Could you check a few things on this model? Use its own coordinates, in mm. Face numbers are marked on the shaded views. A direction names the side the tool comes from. Coordinates: 2 decimals unless noted, no trailing zeros. Order: outer loops, then holes, each group sorted by start corner. A loop starts at its lowest first (then second) coordinate and runs counter-clockwise, first axis right, second up.
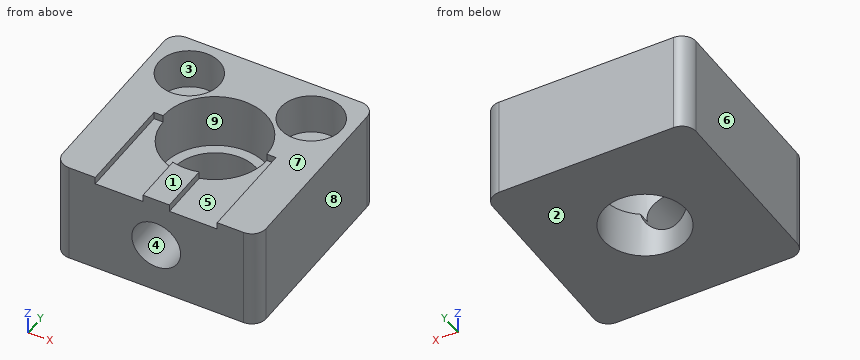
```python
from build123d import *

# Parameters (mm, degrees)
SKETCH1_W           = 10
SKETCH1_H           = 5
BOSS_EXTRUDE1_DEPTH = 10
SKETCH2_R           = 2.05
CUT_EXTRUDE1_DEPTH  = 16
SKETCH3_R           = 2.55
CUT_EXTRUDE2_DEPTH  = 2.7
SKETCH5_W           = 2.35
SKETCH5_H           = 0.35
CUT_EXTRUDE3_DEPTH  = 5
SKETCH6_R           = 1.5
CUT_EXTRUDE4_DEPTH  = 2
SKETCH8_R           = 1.2
CUT_EXTRUDE5_DEPTH  = 3.5
FILLET1_R           = 0.7


with BuildPart() as part:
    # Sketch1 → Boss-Extrude1 (new body)
    with BuildSketch(Plane(origin=(0, 0, 0), x_dir=(1, 0, 0), z_dir=(0, 1, 0))):
        with Locations((5, 2.5)):
            Rectangle(SKETCH1_W, SKETCH1_H)
    extrude(amount=BOSS_EXTRUDE1_DEPTH)

    # Sketch2 → Cut-Extrude1 (cut, through all)
    with BuildSketch(Plane.XY):
        with Locations((5, 5)):
            Circle(SKETCH2_R)
    extrude(amount=-CUT_EXTRUDE1_DEPTH, mode=Mode.SUBTRACT)

    # Sketch3 → Cut-Extrude2 (cut)
    with BuildSketch(Plane.XY):
        with Locations((5, 5)):
            Circle(SKETCH3_R)
    extrude(amount=-CUT_EXTRUDE2_DEPTH, mode=Mode.SUBTRACT)

    # Sketch5 → Cut-Extrude3 (cut)
    with BuildSketch(Plane.XZ):
        with Locations((3.175, -0.175)):
            Rectangle(SKETCH5_W, SKETCH5_H)
        with Locations((6.825, -0.175)):
            Rectangle(SKETCH5_W, SKETCH5_H)
    extrude(amount=-CUT_EXTRUDE3_DEPTH, mode=Mode.SUBTRACT)

    # Sketch6 → Cut-Extrude4 (cut)
    with BuildSketch(Plane.XY):
        with Locations((2, 8)):
            Circle(SKETCH6_R)
        with Locations((8, 8)):
            Circle(SKETCH6_R)
    extrude(amount=-CUT_EXTRUDE4_DEPTH, mode=Mode.SUBTRACT)

    # Sketch8 → Cut-Extrude5 (cut)
    with BuildSketch(Plane.XZ):
        with Locations(Location((5, -2.5, 0), (0, 0, 270))):
            Circle(SKETCH8_R)
    extrude(amount=-CUT_EXTRUDE5_DEPTH, mode=Mode.SUBTRACT)

    # Fillet1
    fillet1_edges = [part.edges().sort_by_distance(p)[0] for p in [
        (10, 10, -2.5),
        (0, 10, -2.5),
        (10, 0, -2.5),
        (0, 0, -2.5),
    ]]
    fillet(fillet1_edges, radius=FILLET1_R)


solid = part.part
```
Item 1: Suppose I cut it at B-B (y = 4.5). List the corners of the cut face in (x, z) for me.
Item 2: Suppose I cut it at D-D (y = 8). List the corners of the cut face in (x, z) for me.
Item 3: Which directions (+Z, -Z, +X, -X, +Y, -Y) give clear straight access to the entire face, cutting with the end or side of a thin tool? Please do the marked faces 1, 2, 3, 4 and 5.
Item 4: I need wall thicknesses on line 1 (Y direction, x = 5, z = -1.2); line 2 (Y direction, x = 2, z = -0.75); line 3 (X direction, y = 5, z = -4.1). Which ranges of each line are inside material? Lowest first, please.
Item 5: Suppose I cut it at C-C (z = -2.5). List the corners of the cut face in (x, y) for me.
Item 6: Suppose I cut it at A-A (x = 5). List the corners of the cut face in (y, z) for me, and give its area (3 significant figures).
Item 7: Thinking about a two-plate mould opening in X: for the marked faces 6, 7, 8 and 9, which applies, +X half, -X half, draft (parallel to the pull), parting line (faces both ways), or undercut?
Item 8: For pin 1 Ø3.5 at (x, y) = (2, 8) entering from +Z; pin 2 Ø0.9 at (x, y) = (7.5, 8.5) entering from +Z; pin 3 Ø1.9 at (x, y) = (3, 2.5) entering from +Z; pin 4 Ø2.5 at (x, y) = (4, 5) entering from +Z, each with a flat end and sliding along its axis, tell me the tip position at first contact or that it passes through.
Geometry results:
1. outline: (0, -5) - (3.01, -5) - (3.01, -2.7) - (2.5, -2.7) - (2.5, -0.35) - (2, -0.35) - (2, 0) - (0, 0) - close; (6.99, -5) - (10, -5) - (10, 0) - (8, 0) - (8, -0.35) - (7.5, -0.35) - (7.5, -2.7) - (6.99, -2.7) - close
2. outline: (0, -5) - (10, -5) - (10, 0) - (9.5, 0) - (9.5, -2) - (6.5, -2) - (6.5, 0) - (3.5, 0) - (3.5, -2) - (0.5, -2) - (0.5, 0) - (0, 0) - close
3. face 1: +Z, +X, -X, +Y, -Y
3. face 2: -Z, +X, -X, +Y, -Y
3. face 3: +Z
3. face 4: -Y
3. face 5: +Z, -Y
4. line 1: y = 0 to 2.45, 7.55 to 10
4. line 2: y = 0 to 6.5, 9.5 to 10
4. line 3: x = 0 to 2.95, 7.05 to 10
5. outline: (0, 0.7) arc R0.7 ccw to (0.7, 0) - (3.8, 0) - (3.8, 2.75) arc R2.55 cw (long way) to (6.2, 2.75) - (6.2, 0) - (9.3, 0) arc R0.7 ccw to (10, 0.7) - (10, 9.3) arc R0.7 ccw to (9.3, 10) - (0.7, 10) arc R0.7 ccw to (0, 9.3) - close
6. outline: (0, -5) - (2.95, -5) - (2.95, -3.7) - (0, -3.7) - close; (0, -1.3) - (2.45, -1.3) - (2.45, 0) - (0, 0) - close; (7.05, -5) - (10, -5) - (10, 0) - (7.55, 0) - (7.55, -2.7) - (7.05, -2.7) - close
6. area: 20.4 mm2
7. face 6: -X half
7. face 7: draft
7. face 8: +X half
7. face 9: undercut
8. pin 1: stops at z = 0
8. pin 2: stops at z = -2
8. pin 3: stops at z = -0.35
8. pin 4: stops at z = -2.7
